Verification items for the finished model (mm, model axes). A direction names the side the tool comes from. Round coordinates to 2 decimals unless told otherwise and drop trailing zeros. Write each loop counter-clockwise with the first axis right and the second up, starting at its lowest first coordinate (ties: lowest second). Pieces come first, ordered by that corner, then holes. Notation, with made-up numbers: M -24.75,14 L -3.75,14 A16 cw -3.75,25 Z; hole C 6,-30 d3. An arc over 180 degrees is marked long. One line per question, with ' | ' between items.
from build123d import *
from build123d.topology import SkipClean

# Parameters (mm, degrees)
SKETCH1_R           = 1.075
BOSS_EXTRUDE1_DEPTH = 6
CUT_EXTRUDE1_START  = -2
CUT_EXTRUDE1_DEPTH  = 2
CUT_EXTRUDE2_DEPTH  = 2


with BuildPart() as part:
    # Sketch1 → Boss-Extrude1 (new body)
    with BuildSketch(Plane(origin=(0, 0, 0), x_dir=(1, 0, 0), z_dir=(0, 1, 0))):
        with BuildLine():
            Line((0, 2), (7.5, 2))
            ThreePointArc((7.5, 2), (9.5, 0), (7.5, -2))
            Line((7.5, -2), (0, -2))
            ThreePointArc((0, -2), (-2, 0), (0, 2))
        make_face()
        with Locations(Location((0, 0, 0), (0, 0, 270))):
            Circle(SKETCH1_R, mode=Mode.SUBTRACT)
        with Locations(Location((7.5, 0, 0), (0, 0, 270))):
            Circle(SKETCH1_R, mode=Mode.SUBTRACT)
    extrude(amount=BOSS_EXTRUDE1_DEPTH)

    # Sketch2 → Cut-Extrude1 (cut)
    with BuildSketch(Plane(origin=(0, 6, 0), x_dir=(1, 0, 0), z_dir=(0, 1, 0)).offset(CUT_EXTRUDE1_START)):
        with BuildLine():
            Line((0, 2), (7.5, 2))
            ThreePointArc((7.5, 2), (5.5, 0), (7.5, -2))
            Line((7.5, -2), (0, -2))
            ThreePointArc((0, -2), (-2, 0), (0, 2))
        make_face()
    extrude(amount=CUT_EXTRUDE1_DEPTH, mode=Mode.SUBTRACT)

    # Sketch3 → Cut-Extrude2 (cut)
    with SkipClean():  # the faces are left unmerged after this step: merging them gives an invalid solid
        with BuildSketch(Plane.XZ):
            with BuildLine():
                Line((7.5, 2), (0, 2))
                ThreePointArc((0, 2), (2, 0), (0, -2))
                Line((0, -2), (7.5, -2))
                ThreePointArc((7.5, -2), (9.5, 0), (7.5, 2))
            make_face()
        extrude(amount=-CUT_EXTRUDE2_DEPTH, mode=Mode.SUBTRACT)


solid = part.part
1. Thickness scan on line 1 (X direction, y = 3.95, z = 0) (3 decimals); line 2 (X direction, y = 1.95, z = 0) (3 decimals); line 3 (X direction, y = 4.5, z = 0) (3 decimals). Record the ranges inside material, lowest first.
Results:
line 1: x = -2 to -1.075, 1.075 to 6.425, 8.575 to 9.5 | line 2: x = -2 to -1.075, 1.075 to 2 | line 3: x = 5.5 to 6.425, 8.575 to 9.5
2. Go/stop test with flat-tipped pins: P1, Ø1.3, axis at x = 7.5, z = 0, coming from the -Y side; P2, Ø1, axis at y = 1, z = 1, coming from the -X side; P3, Ø1, axis at x = 3, z = 1, coming from the -Y side. Record where each tip stops, or that it passes through.
Results:
P1: passes through | P2: stops at x = -1.94 | P3: stops at y = 2
3. Section check B-B, the plane x = -0.5. Record the cut outline in (y, z), then the cut area to 3 significant figures.
Results:
outline: M 0,-1.94 L 4,-1.94 L 4,-0.95 L 0,-0.95 Z; M 0,0.95 L 4,0.95 L 4,1.94 L 0,1.94 Z | area: 7.88 mm2
4. Tool access check on faces 1 (the face through (-1, 0, 1)), 2 (the face through (9.483, 4.416, 0.26)). Record the directions out of +Z, -Z, +X, -X, +Y, -Y that give a thin tool (end or side, any length) a straight path to the whole face; none if there is none.
Results:
face 1: +Z, -Z, +X, -X, -Y | face 2: +Y
5. Section check A-A, the plane z = 0. Record the cut outline in (x, y) (3 decimals), then the cut area to 3 significant figures.
Results:
outline: M -2,0 L -1.075,0 L -1.075,4 L -2,4 Z; M 1.075,0 L 2,0 L 2,2 L 6.425,2 L 6.425,6 L 5.5,6 L 5.5,4 L 1.075,4 Z; M 8.575,2 L 9.5,2 L 9.5,6 L 8.575,6 Z | area: 21.8 mm2
6. Section check C-C, the plane z = 0.8. Record the cut outline in (x, y).
Results:
outline: M -1.83,0 L -0.72,0 L -0.72,4 L -1.83,4 Z; M 0.72,0 L 1.83,0 L 1.83,2 L 6.78,2 L 6.78,6 L 5.67,6 L 5.67,4 L 0.72,4 Z; M 8.22,2 L 9.33,2 L 9.33,6 L 8.22,6 Z
7. Section check D-D, the plane y = 5.1. Record the cut outline in (x, z) (3 decimals), then the cut area to 3 significant figures.
Results:
outline: C 7.5,0 d4; hole C 7.5,0 d2.15 | area: 8.94 mm2
8. Mould release check, pull along X, two halves, no side actions. Record for faces 3 (the face through (6.45, 3.97, -0.23)), 4 (the face through (-2, 2, 0)), 5 (the face through (4, 3, -2)): pulls with the +X half, pulls with the -X half, needs draft (parallel to the pull), parting line crosses it, or undercut.
Results:
face 3: undercut | face 4: parting line crosses it | face 5: needs draft
